Input: part model. Units: mm. Frame: model coordinates. A direction names the side the tool comes from. Coordinates: 2 decimals unless noted, no trailing zeros. Loops run counter-clockwise (first coordinate to the right, second up) from the corner with the lowest first, then second, coordinate; pieces in that order, holes last.
Item 1: Section B-B on x = 2. Return loops of the section in (y, z).
Item 2: Contact query for flat-ended pins moving along their axis: P1, Ø3, axis at x = -2, z = -5, coming from the -Y side; P2, Ø10, axis at x = 5.5, z = -8, coming from the +Y side. Output: stop coordinate, or through.
Item 3: Section C-C on y = 142. Return loops of the section in (x, z), and give its area (3 significant figures).
Item 4: Ray query, line 1 along Z through (x, y) = (-1.25, 153); line 2 along Z through (x, y) = (-7.5, -70.5). Return the intervals inside material, ascending.
Item 5: Reachability of faces 4 (the flat face through (-8, -3, 0)), 5 (the flat face through (0, -3, 10)) from +Z, -Z, +X, -X, +Y, -Y: full face, straight path, thin tool, end or side. Return the list, or none.
Item 6: Pull-direction query (Z, two-part tool) for faces 1 (the flat face through (8, -3, 0)), 2 (the flat face through (-10, -3, 0)), 3 (the flat face through (9, 180, 0)); classes: released by +Z, released by -Z, zero draft, split by the parting line, or undercut.
Item 7: Section A-A on z = 2.25. Return loops of the section in (x, y), and give its area (3 significant figures).
```python
from build123d import *

# Parameters (mm, degrees)
F2_W     = 20
F2_H     = 20
F3_DEPTH = 190
F4_R     = 3
F5_T     = -2
F7_DEPTH = 20.001
F9_DEPTH = 20.001


with BuildPart() as f3:
    # F2 (on Front) → F3 (new body, symmetric)
    with BuildSketch(Plane.XZ):
        Rectangle(F2_W, F2_H)
    extrude(amount=F3_DEPTH, both=True)

    # F4
    f4_edges = [f3.edges().sort_by_distance(p)[0] for p in [
        (10, 0, 10),
        (-10, 0, 10),
        (10, 0, -10),
        (-10, 0, -10),
    ]]
    fillet(f4_edges, radius=F4_R)

    # F5
    f5_openings = [f3.faces().sort_by_distance(p)[0] for p in [
        (0, -190, 0),
        (0, 190, 0),
    ]]
    offset(amount=F5_T, openings=f5_openings)

    # F6 (on face) → F7 (cut, through all)
    with BuildSketch(Plane(origin=(-10, 0, 0), x_dir=(0, -1, 0), z_dir=(-1, 0, 0))):
        Polygon((-190, 10), (-190, -10), (-170, -10), align=None)
    extrude(amount=-F7_DEPTH, mode=Mode.SUBTRACT)

    # F8 (on face) → F9 (cut, through all)
    with BuildSketch(Plane.YZ.offset(10)):
        Polygon((-190, -10), (-170, -10), (-190, 10), align=None)
    extrude(amount=-F9_DEPTH, mode=Mode.SUBTRACT)


solid = f3.part
```
Results found:
1. outline: (-190, 10) - (-188, 8) - (188, 8) - (190, 10) - close; (-172, -8) - (-170, -10) - (170, -10) - (172, -8) - close
2. P1: passes through
2. P2: stops at y = 176.33
3. outline: (-10, -7) arc R3 ccw to (-7, -10) - (7, -10) arc R3 ccw to (10, -7) - (10, 7) arc R3 ccw to (7, 10) - (-7, 10) arc R3 ccw to (-10, 7) - close; hole (-8, -7) arc R1 ccw to (-7, -8) - (7, -8) arc R1 ccw to (8, -7) - (8, 7) arc R1 ccw to (7, 8) - (-7, 8) arc R1 ccw to (-8, 7) - close
3. area: 137 mm2
4. line 1: z = -10 to -8, 8 to 10
4. line 2: z = -9.96 to -7.87, 7.87 to 9.96
5. face 4: +Y, -Y
5. face 5: +Z, +X, -X, +Y, -Y
6. face 1: undercut
6. face 2: zero draft
6. face 3: released by -Z
7. outline: (-10, -182.25) - (-8, -182.25) - (-8, 182.25) - (-10, 182.25) - close; (8, -182.25) - (10, -182.25) - (10, 182.25) - (8, 182.25) - close
7. area: 1,460 mm2
